Part print with two shaded views. Sizes in mm from the minimum x, y, z corner. Round coordinates to 2 decimals unless told otherwise and drop trailing zeros. Write each loop counter-clockwise with the first axis right and the second up, starting at its lowest first coordinate (ties: lowest second). Pieces come first, ordered by that corner, then holes. Notation, with made-up numbers: (73, 14) -> (80, 14) arc R11 cw to (80, 28) -> close; hole circle Ø6 at (57, -35). An arc over 180 degrees is marked (long way). Return JSON: item names as keys, results as strings.
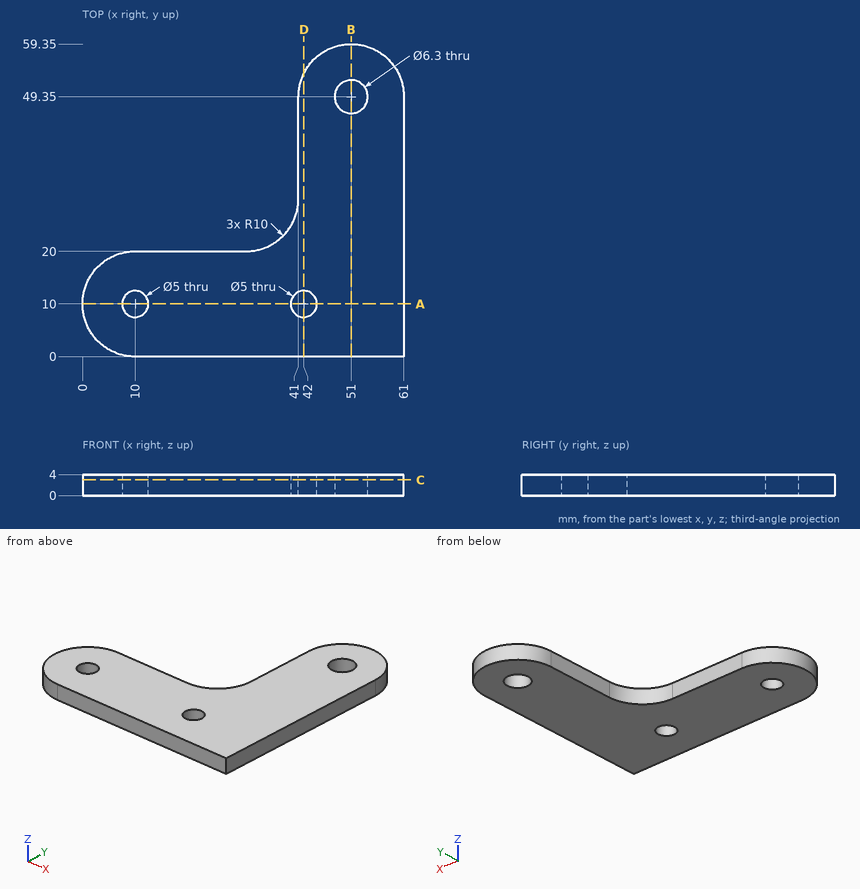
Q1. Pin check, flat tips, straight feed: pin 1 Ø2 at (x, z) = (17.5, 2) entering from +Y; pin 2 Ø5 at (x, y) = (51, 49.35) entering from +Z. Stop position of each tip, or through.
Verdict:
{"pin 1": "stops at y = 20", "pin 2": "passes through"}
Q2. Wall check: L1, parallel to X at y = 44, z = 2.4; L2, parallel to Y at x = 42, z = 1.5; L3, parallel to X at y = 10.5, z = 0.75. Give the ranges that are in metal, low to high.
Verdict:
{"L1": "x = 41 to 61", "L2": "y = 0 to 7.5, 12.5 to 53.71", "L3": "x = 0.01 to 7.55, 12.45 to 39.55, 44.45 to 61"}
Q3. Saw through at B-B on x = 51. List the corners of the cut face in (y, z), then the cut area to 3 significant figures.
Verdict:
{"outline": "(0, 0) -> (46.2, 0) -> (46.2, 4) -> (0, 4) -> close; (52.5, 0) -> (59.35, 0) -> (59.35, 4) -> (52.5, 4) -> close", "area": "212 mm²"}
Q4. Saw through at A-A on y = 10. List the corners of the cut face in (x, z), then the cut area to 3 significant figures.
Verdict:
{"outline": "(0, 0) -> (7.5, 0) -> (7.5, 4) -> (0, 4) -> close; (12.5, 0) -> (39.5, 0) -> (39.5, 4) -> (12.5, 4) -> close; (44.5, 0) -> (61, 0) -> (61, 4) -> (44.5, 4) -> close", "area": "204 mm²"}
Q5. Saw through at C-C on z = 3. List the corners of the cut face in (x, y).
Verdict:
{"outline": "(10, 0) -> (61, 0) -> (61, 49.35) arc R10 ccw to (41, 49.35) -> (41, 30) arc R10 cw to (31, 20) -> (10, 20) arc R10 ccw to start; hole circle Ø5 at (10, 10); hole circle Ø5 at (42, 10); hole circle Ø6.3 at (51, 49.35)"}
Q6. Saw through at D-D on x = 42. List the corners of the cut face in (y, z), then the cut area to 3 significant figures.
Verdict:
{"outline": "(0, 0) -> (7.5, 0) -> (7.5, 4) -> (0, 4) -> close; (12.5, 0) -> (53.71, 0) -> (53.71, 4) -> (12.5, 4) -> close", "area": "195 mm²"}
